For this review, take the finished solid that the model builds, in its own axes (mm). A direction names the side the tool comes from. Round coordinates to 2 decimals unless told otherwise and drop trailing zeros. Write each loop counter-clockwise with the first axis right and the second up, starting at its lowest first coordinate (ties: lowest second). Pieces come first, ordered by that corner, then holes. Notation, with made-up numbers: (-10, 72) -> (8, 72) arc R18 ccw to (8, 99) -> close; hole circle Ø10 at (86, 0.5). An arc over 180 degrees is marked (long way). Answer as CSV lines item,"result". Start each with the question number.
Item 1: Take a section at C-C on y = -15. Give the boundary of the cut face in (x, z), then the cut area to 3 significant figures.
Item 2: Take a section at A-A on z = 77. Give the boundary of the cut face in (x, y), then the cut area to 3 significant figures.
Item 3: Machinability: for faces 1 (the flat face through (-110, 82.518, 64)), 2 (the cylindrical face through (77.354, 83.532, 1.426)), 3 (the flat face through (75, 82.518, 79)), 4 (the flat face through (-119, 84.518, 79)), which of the approach directions +Z, -Z, +X, -X, +Y, -Y give a long, thin tool a straight path to every point of the face, cutting with its end or side? Answer none if there is none.
Item 4: Mouldability with a two-part tool opening along X and no side actions: class faces 5 (the cylindrical face through (-105.156, 98.014, 1.426)), 6 (the flat face through (68.858, 12, 79)), 7 (the flat face through (-129.142, 14, 81)), 8 (the flat face through (-106.142, 93, 79)) as +X half, -X half, draft (parallel to the pull), parting line (faces both ways), or undercut.
Item 5: Take a section at B-B on x = 36. Give the boundary of the cut face in (y, z), then the cut area to 3 significant figures.
Item 6: Wall thickness on probe 1 along X at (y, z) = (-42, 124); probe 2 along X at (y, z) = (84, 121); probe 3 along Y at (x, z) = (-112, 127.5): over which ranges is each line inside the solid? List them lowest first. Write a range as from..to.
Item 7: For pin 1 Ø4 at (y, z) = (90.5, 108.5) entering from -X; pin 2 Ø8.5 at (y, z) = (90.5, 47) entering from +X; pin 3 Ø10 at (x, y) = (-27, 18.5) entering from +Z, all flat-tipped, find the tip position at first contact; note any pin that passes through.
```python
from build123d import *

# Parameters (mm, degrees)
F0_W     = 10
F0_H     = 2
F1_DEPTH = 160
F0_W_2   = 171
F2_DEPTH = 7
F3_DEPTH = 2
F4_R     = 5
F5_R     = 2


with BuildPart() as f1:
    # F0 (on Top) → F1 (new body)
    with BuildSketch(Plane.XY):
        Polygon((-106.142494, 84.517702), (-131.142494, 84.517702), (-131.142494, -55.482298), (68.857506, -55.482298), (68.857506, 82.517702), (68.857506, 84.517702), (66.857506, 84.517702), (66.857506, 82.517702), (66.857506, -53.482298), (-129.142494, -53.482298), (-129.142494, 82.517702), (-104.142494, 82.517702), (-104.142494, 84.517702), (-104.142494, 99.517702), (-106.142494, 99.517702), align=None)
        with Locations((73.857506, 83.517702)):
            Rectangle(F0_W, F0_H)
    extrude(amount=F1_DEPTH)

    # F0 (on Top) → F2 (join)
    with BuildSketch(Plane.XY):
        with Locations((-18.642494, 83.517702)):
            Rectangle(F0_W_2, F0_H)
    extrude(amount=F2_DEPTH)

    # F0 (on Top) → F3 (join)
    with BuildSketch(Plane.XY):
        Polygon((66.857506, 82.517702), (-104.142494, 82.517702), (-129.142494, 82.517702), (-129.142494, -53.482298), (66.857506, -53.482298), align=None)
    extrude(amount=F3_DEPTH)

    # F4
    f4_edges = [f1.edges().sort_by_distance(p)[0] for p in [
        (-105.142494, 99.517702, 160),
        (-105.142494, 99.517702, 0),
        (78.857506, 83.517702, 0),
        (78.857506, 83.517702, 160),
    ]]
    fillet(f4_edges, radius=F4_R)

    # F5
    f5_edges = [f1.edges().sort_by_distance(p)[0] for p in [
        (-129.142494, -53.482298, 81),
        (-31.142494, -53.482298, 2),
        (-129.142494, 14.517702, 2),
        (66.857506, 14.517702, 2),
        (66.857506, -53.482298, 81),
        (-129.142494, 82.517702, 81),
        (-31.142494, 82.517702, 2),
        (68.857506, 82.517702, 80),
        (-106.142494, 84.517702, 80),
    ]]
    fillet(f5_edges, radius=F5_R)


solid = f1.part
```
Output values:
1,outline,"(-131.14, 0) -> (68.86, 0) -> (68.86, 160) -> (66.86, 160) -> (66.86, 4) arc R2 cw to (64.86, 2) -> (-127.14, 2) arc R2 cw to (-129.14, 4) -> (-129.14, 160) -> (-131.14, 160) -> close"
1,area,"1,030 mm^2"
2,outline,"(-131.14, -55.48) -> (68.86, -55.48) -> (68.86, 80.52) arc R2 cw to (70.86, 82.52) -> (78.86, 82.52) -> (78.86, 84.52) -> (66.86, 84.52) -> (66.86, -51.48) arc R2 cw to (64.86, -53.48) -> (-127.14, -53.48) arc R2 cw to (-129.14, -51.48) -> (-129.14, 80.52) arc R2 cw to (-127.14, 82.52) -> (-104.14, 82.52) -> (-104.14, 99.52) -> (-106.14, 99.52) -> (-106.14, 86.52) arc R2 cw to (-108.14, 84.52) -> (-131.14, 84.52) -> close"
2,area,"1,060 mm^2"
3,face 1,"+Z"
3,face 2,"-Z, +X, +Y, -Y"
3,face 3,"+Z, -Z, +X, -Y"
3,face 4,"+Z, -Z, -X, +Y"
4,face 5,"draft"
4,face 6,"+X half"
4,face 7,"undercut"
4,face 8,"-X half"
5,outline,"(-55.48, 0) -> (84.52, 0) -> (84.52, 7) -> (82.52, 7) -> (82.52, 4) arc R2 cw to (80.52, 2) -> (-51.48, 2) arc R2 cw to (-53.48, 4) -> (-53.48, 160) -> (-55.48, 160) -> close"
5,area,"608 mm^2"
6,probe 1,"x = -131.14..-129.14, 66.86..68.86"
6,probe 2,"x = -131.14..-104.14, 66.86..78.86"
6,probe 3,"y = -55.48..-53.48, 82.52..84.52"
7,pin 1,"stops at x = -106.14"
7,pin 2,"stops at x = -104.14"
7,pin 3,"stops at z = 2"
